from build123d import *

# Parameters (mm, degrees)
F1_DEPTH = 25
F2_T     = 3


# Not quite as in the source:
# - a shell that OpenCascade refuses in one call is made with other operations: the cavity is built on its own and cut out


with BuildPart() as f1:
    # F0 (on Front) → F1 (new body)
    with BuildSketch(Plane.XZ):
        with BuildLine():
            Line((-30.3064525574, 35.3830642998), (-55.4274195135, 35.3830642998))
            ThreePointArc((-55.4274195135, 35.3830642998), (-57.548739857, 34.5043846434), (-58.4274195135, 32.3830642998))
            Line((-58.4274195135, 32.3830642998), (-58.4274195135, 23.8669360727))
            ThreePointArc((-58.4274195135, 23.8669360727), (-57.548739857, 21.7456157291), (-55.4274195135, 20.8669360727))
            Line((-55.4274195135, 20.8669360727), (-30.3064525574, 20.8669360727))
            ThreePointArc((-30.3064525574, 20.8669360727), (-28.1851322139, 21.7456157291), (-27.3064525574, 23.8669360727))
            Line((-27.3064525574, 23.8669360727), (-27.3064525574, 32.3830642998))
            ThreePointArc((-27.3064525574, 32.3830642998), (-28.1851322139, 34.5043846434), (-30.3064525574, 35.3830642998))
        make_face()
    extrude(amount=F1_DEPTH)

    # F2: shell of thickness 3, made by hand


with BuildPart() as f2_core1:
    # F2_t2: copy of F1
    add(f1.part)

    # the walls: a layer under each face that stays
    f2_faces = [f2_core1.faces().sort_by_distance(p)[0] for p in [
        (-42.8669360355, -12.5, 35.3830642998),
        (-58.4274195135, -12.5, 28.1250001863),
        (-42.8669360355, -12.5, 20.8669360727),
        (-27.3064525574, -12.5, 28.1250001863),
        (-42.8669360355, 0, 28.1250001863),
    ]]
    thicken(f2_faces, amount=-F2_T, mode=Mode.SUBTRACT)


with BuildPart() as f1_1:
    add(f1.part)

    # what is left inside the walls is the cavity
    f2_cavity = [f2_core1.part.solids().sort_by_distance(p)[0] for p in [
        (-42.866936, -17.666667, 23.896936),
    ]]
    add(f2_cavity, mode=Mode.SUBTRACT)


solid = f1_1.part
Design review of the part built by this model. Coordinates are the model's own, in mm. A direction names the side the tool comes from. Coordinates: 2 decimals unless noted, no trailing zeros. Loops run counter-clockwise (first coordinate to the right, second up) from the corner with the lowest first, then second, coordinate; pieces in that order, holes last.
Item 1: Add section C-C (y = -21.5). Write out the cut boundary in (x, z), and give its area (3 significant figures).
Completed:
outline: (-58.43, 23.87) arc R3 ccw to (-55.43, 20.87) - (-30.31, 20.87) arc R3 ccw to (-27.31, 23.87) - (-27.31, 32.38) arc R3 ccw to (-30.31, 35.38) - (-55.43, 35.38) arc R3 ccw to (-58.43, 32.38) - close; hole (-55.43, 23.87) - (-30.31, 23.87) - (-30.31, 32.38) - (-55.43, 32.38) - close
area: 230 mm2
Item 2: For faces 5 (the flat face through (-55.427, -14, 28)), 6 (the cylindrical face through (-57.6, -12.3, 21.8)), list the 3-axis set-ups (+Z, -Z, +X, -X, +Y, -Y) from which the entire face can be reached by the end or side of a thin tool; tool diameter is ignored.
Completed:
face 5: -Y
face 6: -Z, -X, +Y, -Y
Item 3: Add section D-D (z = 22.5). Write out the cut boundary in (x, y).
Completed:
outline: (-58.1, -25) - (-27.64, -25) - (-27.64, 0) - (-58.1, 0) - close
Item 4: Wall thickness on L1, parallel to Z at x = -42.5, y = -20; L2, parallel to X at y = -12, z = 26.5; L3, parallel to Y at x = -45.5, z = 27: over which ranges is each line inside the solid? List them lowest first.
Completed:
L1: z = 20.87 to 23.87, 32.38 to 35.38
L2: x = -58.43 to -55.43, -30.31 to -27.31
L3: y = -3 to 0
Item 5: Draft analysis for pull direction X (two halves, no side actions). For faces 1 (the flat face through (-43, -25, 33)), 2 (the flat face through (-43, -14, 23.867)), 3 (the cylindrical face through (-28.21, -12.32, 21.72)), 4 (the flat face through (-30.306, -14, 28)), state which applies: pulls with the +X half, pulls with the -X half, needs draft (parallel to the pull), parting line crosses it, or undercut.
Completed:
face 1: needs draft
face 2: undercut
face 3: pulls with the +X half
face 4: undercut
Item 6: Add section B-B (z = 27.5). Write out the cut boundary in (x, y), and give its area (3 significant figures).
Completed:
outline: (-58.43, -25) - (-55.43, -25) - (-55.43, -3) - (-30.31, -3) - (-30.31, -25) - (-27.31, -25) - (-27.31, 0) - (-58.43, 0) - close
area: 225 mm2
Item 7: Add section A-A (y = -1.75). Write out the cut boundary in (x, z), and give its area (3 significant figures).
Completed:
outline: (-58.43, 23.87) arc R3 ccw to (-55.43, 20.87) - (-30.31, 20.87) arc R3 ccw to (-27.31, 23.87) - (-27.31, 32.38) arc R3 ccw to (-30.31, 35.38) - (-55.43, 35.38) arc R3 ccw to (-58.43, 32.38) - close
area: 444 mm2
